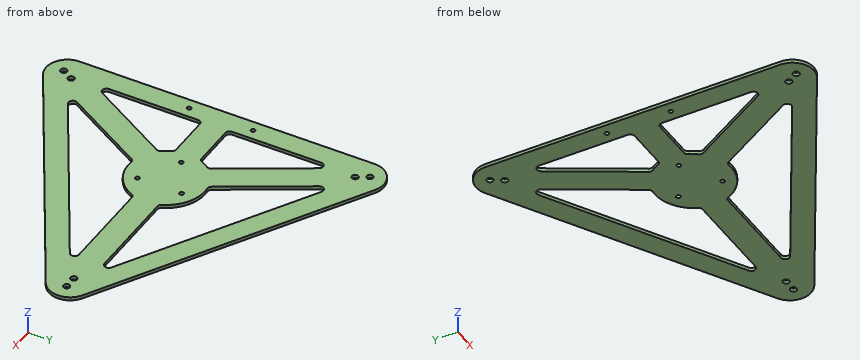
from build123d import *

# Parameters (mm, degrees)
BOARD_DEPTH     = 0.8
CUT_DEPTH       = 60.975412975
HOLESSKE_R      = 0.5
HOLES_DEPTH     = 60.975412975
HOLES2SKE_R     = 0.75
HOLES2_DEPTH    = 60.975412975
HOLES3SKE_R     = 0.5
HOLES3_DEPTH    = 60.975412975
REINFORCE_START = 0.8
REINFORCE_DEPTH = 0.8


with BuildPart() as part:
    # BoardSke → Board (new body)
    with BuildSketch(Plane.XY):
        with BuildLine():
            Line((42.5, 4.330127019), (-17.5, 38.97114317))
            ThreePointArc((-17.5, 38.97114317), (-22.5, 38.97114317), (-25, 34.641016151))
            Line((-25, 34.641016151), (-25, -34.641016151))
            ThreePointArc((-25, -34.641016151), (-22.5, -38.97114317), (-17.5, -38.97114317))
            Line((-17.5, -38.97114317), (42.5, -4.330127019))
            ThreePointArc((42.5, -4.330127019), (45, 0), (42.5, 4.330127019))
        make_face()
    extrude(amount=BOARD_DEPTH)

    # CutSke → Cut (cut, through all)
    with BuildSketch(Plane.XY.offset(0.8)):
        with BuildLine():
            Line((31.07179677, 3), (9.16515139, 3))
            ThreePointArc((9.16515139, 3), (8.617428832, 3.163339973), (8.248636251, 3.6))
            ThreePointArc((8.248636251, 3.6), (4.5, 7.794228634), (-1.006626672, 8.94352854))
            ThreePointArc((-1.006626672, 8.94352854), (-1.569181638, 9.044582271), (-1.984499484, 9.437253933))
            Line((-1.984499484, 9.437253933), (-12.937822174, 28.408965344))
            ThreePointArc((-12.937822174, 28.408965344), (-12.778903551, 29.616072125), (-11.57179677, 29.774990748))
            Line((-11.57179677, 29.774990748), (31.57179677, 4.866025404))
            ThreePointArc((31.57179677, 4.866025404), (32.037722596, 3.741180955), (31.07179677, 3))
        make_face()
        with BuildLine():
            Line((31.07179677, -3), (9.16515139, -3))
            ThreePointArc((9.16515139, -3), (8.617428832, -3.163339973), (8.248636251, -3.6))
            ThreePointArc((8.248636251, -3.6), (4.5, -7.794228634), (-1.006626672, -8.94352854))
            ThreePointArc((-1.006626672, -8.94352854), (-1.569181638, -9.044582271), (-1.984499484, -9.437253933))
            Line((-1.984499484, -9.437253933), (-12.937822174, -28.408965344))
            ThreePointArc((-12.937822174, -28.408965344), (-12.778903551, -29.616072125), (-11.57179677, -29.774990748))
            Line((-11.57179677, -29.774990748), (31.57179677, -4.866025404))
            ThreePointArc((31.57179677, -4.866025404), (32.037722596, -3.741180955), (31.07179677, -3))
        make_face()
        with BuildLine():
            Line((-18.133974596, -25.408965344), (-7.180651906, -6.437253933))
            ThreePointArc((-7.180651906, -6.437253933), (-7.048247194, -5.881242297), (-7.242009579, -5.34352854))
            ThreePointArc((-7.242009579, -5.34352854), (-9, 0), (-7.242009579, 5.34352854))
            ThreePointArc((-7.242009579, 5.34352854), (-7.048247194, 5.881242297), (-7.180651906, 6.437253933))
            Line((-7.180651906, 6.437253933), (-18.133974596, 25.408965344))
            ThreePointArc((-18.133974596, 25.408965344), (-19.258819045, 25.87489117), (-20, 24.908965344))
            Line((-20, 24.908965344), (-20, -24.908965344))
            ThreePointArc((-20, -24.908965344), (-19.258819045, -25.87489117), (-18.133974596, -25.408965344))
        make_face()
    extrude(amount=-CUT_DEPTH, mode=Mode.SUBTRACT)

    # HolesSke → Holes (cut, through all)
    with BuildSketch(Plane.XY.offset(0.8)):
        with Locations((-6, 0)):
            Circle(HOLESSKE_R)
        with Locations((3, 5.196152423)):
            Circle(HOLESSKE_R)
        with Locations((3, -5.196152423)):
            Circle(HOLESSKE_R)
    extrude(amount=-HOLES_DEPTH, mode=Mode.SUBTRACT)

    # Holes2Ske → Holes2 (cut, through all)
    with BuildSketch(Plane.XY.offset(0.8)):
        with Locations((38.5, 0)):
            Circle(HOLES2SKE_R)
        with Locations((41.5, 0)):
            Circle(HOLES2SKE_R)
        with Locations((-19.25, -33.341978046)):
            Circle(HOLES2SKE_R)
        with Locations((-20.75, -35.940054257)):
            Circle(HOLES2SKE_R)
        with Locations((-19.25, 33.341978046)):
            Circle(HOLES2SKE_R)
        with Locations((-20.75, 35.940054257)):
            Circle(HOLES2SKE_R)
    extrude(amount=-HOLES2_DEPTH, mode=Mode.SUBTRACT)

    # Holes3Ske → Holes3 (cut, through all)
    with BuildSketch(Plane.XY.offset(0.8)):
        with Locations((-22.5, 7.5)):
            Circle(HOLES3SKE_R)
        with Locations((-22.5, -7.5)):
            Circle(HOLES3SKE_R)
    extrude(amount=-HOLES3_DEPTH, mode=Mode.SUBTRACT)

    # ReinforceSke → Reinforce (add)
    with BuildSketch(Plane.XY.offset(REINFORCE_START)):
        with BuildLine():
            Line((-9.16515139, 3), (-19, 3))
            ThreePointArc((-19, 3), (-19.707106781, 3.292893219), (-20, 4))
            Line((-20, 4), (-20, -4))
            ThreePointArc((-20, -4), (-19.707106781, -3.292893219), (-19, -3))
            Line((-19, -3), (-9.16515139, -3))
            ThreePointArc((-9.16515139, -3), (-8.617428832, -3.163339973), (-8.248636251, -3.6))
            ThreePointArc((-8.248636251, -3.6), (-9, 0), (-8.248636251, 3.6))
            ThreePointArc((-8.248636251, 3.6), (-8.617428832, 3.163339973), (-9.16515139, 3))
        make_face()
    extrude(amount=-REINFORCE_DEPTH)


solid = part.part
Model file for the job. Use its own axes, mm. Give positions to 0.01 mm unless a question says otherwise; leave off trailing zeros. Write each loop counter-clockwise with the first axis right and the second up, starting at its lowest first coordinate (ties: lowest second). Pieces come first, ordered by that corner, then holes. Notation, with made-up numbers: M -13.75,88.5 L 0.25,88.5 A26 cw 0.25,127.5 Z; hole C -11.75,30 d4. An arc over 180 degrees is marked long. One line per item, written item: value. Start each with the question number.
Q1. Saw through at B-B, the plane y = -11.5. Write the cut outline in (x, z).
Q2. Saw through at C-C, the plane z = 0.4. State how many separate pieces and enclosed holes the cut face has, plus the area to 3 significant figures.
Q3. Probe probe 1 along Y at (x, z) = (-22.5, 0.25); probe 2 along Y at (x, z) = (20.5, 0.4); probe 3 along X at (y, z) = (16.5, 0.75). List the from-to ranges inside material, lowest first. Write a range as [from, to].
Q4. Saw through at A-A, the plane x = 15. Write the cut outline in (y, z).
Output values:
1. outline: M -25,0 L -20,0 L -20,0.8 L -25,0.8 Z; M -10.1,0 L -3.18,0 L -3.18,0.8 L -10.1,0.8 Z; M 20.08,0 L 30.08,0 L 30.08,0.8 L 20.08,0.8 Z
2. separate pieces: 1
2. enclosed holes: 15
2. area: 1,950 mm²
3. probe 1: y = [-38.97, -8], [-7, 7], [8, 38.97]
3. probe 2: y = [-17.03, -11.26], [-3, 3], [11.26, 17.03]
3. probe 3: x = [-25, -20], [-12.99, -6.06], [11.42, 21.42]
4. outline: M -20.21,0 L -14.43,0 L -14.43,0.8 L -20.21,0.8 Z; M -3,0 L 3,0 L 3,0.8 L -3,0.8 Z; M 14.43,0 L 20.21,0 L 20.21,0.8 L 14.43,0.8 Z
